Design review of the part built by this model. Coordinates are the model's own, in mm. Face numbers are marked on the shaded views. A direction names the side the tool comes from. Give positions to 0.01 mm unless a question says otherwise; leave off trailing zeros. Write each loop counter-clockwise with the first axis right and the second up, starting at its lowest first coordinate (ties: lowest second). Pieces come first, ordered by that corner, then holes. Notation, with made-up numbers: (71.5, 31) -> (129.5, 31) arc R14 ccw to (129.5, 45) -> close; hole circle Ø7 at (-13, 36.25). An arc over 180 degrees is marked (long way). Answer as a JSON object with one key per item and string values.
```python
from build123d import *

# Parameters (mm, degrees)
SKETCH1_R           = 1.65
BOSS_EXTRUDE1_DEPTH = 5
FILLET2_R           = 0.25
CUT_EXTRUDE1_DEPTH  = 4


with BuildPart() as part:
    # Sketch1 → Boss-Extrude1 (new body)
    # profile 1 of 2: a face of its own
    with BuildSketch(Plane.XY):
        with BuildLine():
            Line((-5.168635154, -1.464478016), (-25.218635154, -1.464478016))
            ThreePointArc((-25.218635154, -1.464478016), (-30.218635154, -6.464478016), (-25.218635154, -11.464478016))
            Line((-25.218635154, -11.464478016), (-3.218635154, -11.464478016))
            Line((-3.218635154, -11.464478016), (1.36555506, -4.468181425))
            ThreePointArc((1.36555506, -4.468181425), (-0.47833252, -2.282284635), (-3.218635154, -1.464478016))
            Line((-3.218635154, -1.464478016), (-5.168635154, -1.464478016))
        make_face()
        with Locations((-25.218635154, -6.464478016)):
            Circle(SKETCH1_R, mode=Mode.SUBTRACT)
        with Locations((-3.197929879, -6.257635448)):
            Circle(SKETCH1_R, mode=Mode.SUBTRACT)
    # profile 2 of 2: a face of its own
    with BuildSketch(Plane.XY):
        with BuildLine():
            Line((35.988446, 15.45724385), (-5.168635154, -1.464478016))
            Line((-5.168635154, -1.464478016), (-3.218635154, -1.464478016))
            ThreePointArc((-3.218635154, -1.464478016), (-0.47833252, -2.282284635), (1.36555506, -4.468181425))
            Line((1.36555506, -4.468181425), (29.450627286, 6.742809526))
            Line((29.450627286, 6.742809526), (35.767904523, 4.15974363))
            Line((35.767904523, 4.15974363), (36.563833051, 3.839605387))
            Line((36.563833051, 3.839605387), (45.016686804, 7.962377757))
            Line((45.016686804, 7.962377757), (43.305501447, 12.124329784))
            Line((43.305501447, 12.124329784), (35.988446, 15.45724385))
        make_face()
    extrude(amount=BOSS_EXTRUDE1_DEPTH)

    # Fillet2
    fillet2_edges = [part.edges().sort_by_distance(p)[0] for p in [
        (-14.218635154, -11.464478016, 0),
        (-30.218635154, -6.464478016, 0),
        (-15.193635154, -1.464478016, 0),
        (15.409905423, 6.996382917, 0),
        (-0.926540047, -7.966329721, 5),
        (39.646973723, 13.790786817, 0),
        (44.161094126, 10.04335377, 0),
        (40.790259928, 5.900991572, 0),
        (36.165868787, 3.999674508, 0),
        (32.609265904, 5.451276578, 0),
        (15.408091173, 1.137314051, 0),
        (-0.926540047, -7.966329721, 0),
        (15.408091173, 1.137314051, 5),
        (-3.218635154, -11.464478016, 2.5),
        (-5.168635154, -1.464478016, 2.5),
        (35.988446, 15.45724385, 2.5),
        (43.305501447, 12.124329784, 2.5),
        (45.016686804, 7.962377757, 2.5),
        (36.563833051, 3.839605387, 2.5),
        (35.767904523, 4.15974363, 2.5),
        (29.450627286, 6.742809526, 2.5),
        (1.36555506, -4.468181425, 2.5),
        (32.609265904, 5.451276578, 5),
        (36.165868787, 3.999674508, 5),
        (40.790259928, 5.900991572, 5),
        (44.161094126, 10.04335377, 5),
        (39.646973723, 13.790786817, 5),
        (15.409905423, 6.996382917, 5),
        (-15.193635154, -1.464478016, 5),
        (-30.218635154, -6.464478016, 5),
        (-14.218635154, -11.464478016, 5),
    ]]
    fillet(fillet2_edges, radius=FILLET2_R)

    # Sketch2 → Cut-Extrude1 (cut)
    with BuildSketch(Plane.XY):
        Polygon((-23.630921913, -9.214478016), (-22.043208673, -6.464478016), (-23.630921913, -3.714478016), (-26.806348394, -3.714478016), (-28.394061634, -6.464478016), (-26.806348394, -9.214478016), align=None)
        Polygon((-0.027560565, -6.436777135), (-1.45760397, -3.601585926), (-4.627973284, -3.422444239), (-6.368299193, -6.078493761), (-4.938255788, -8.91368497), (-1.767886474, -9.092826657), align=None)
    extrude(amount=CUT_EXTRUDE1_DEPTH, mode=Mode.SUBTRACT)


solid = part.part
```
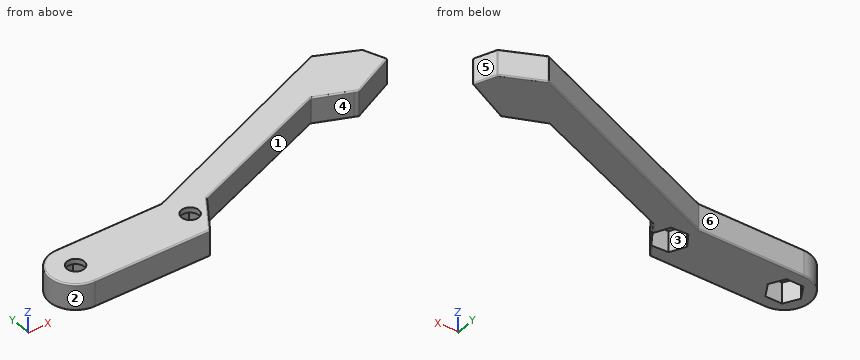
(1) We need section B-B, the plane x = -13. State the section outline as (y, z) points.
Here are the results:
{"outline": "(-11.46, 0.25) arc R0.25 ccw to (-11.21, 0) -> (-1.71, 0) arc R0.25 ccw to (-1.46, 0.25) -> (-1.46, 4.75) arc R0.25 ccw to (-1.71, 5) -> (-11.21, 5) arc R0.25 ccw to (-11.46, 4.75) -> close"}
(2) Clearance check with flat-ended pins moving along their axes: pin 1 (3 mm diameter, centred on x = 18.5, z = 2.5, fed in from -Y); pin 2 (1 mm diameter, centred on x = -25.5, z = 1.5, fed in from +Y). State where each tip first meets the part, or that it passes through.
Here are the results:
{"pin 1": "stops at y = 1.77", "pin 2": "stops at y = -1.46"}
(3) The part is to be moulded in two halves that separate along X. For the marked faces 4, 5 and 6, say which applies: +X half, -X half, draft (parallel to the pull), parting line (faces both ways), or undercut.
Here are the results:
{"face 4": "undercut", "face 5": "+X half", "face 6": "draft"}
(4) We need section A-A, the plane z = 1.8. Give the number of separate pieces and of enclosed holes in the cut face, then the cut area to 3 significant figures.
Here are the results:
{"separate pieces": "1", "enclosed holes": "2", "area": "533 mm²"}
(5) For line 1 along X through (y, z) = (-6.25, 0.3); line 2 along Y through (x, z) = (-15, 4.5); line 3 along Y through (x, z) = (-27, 2.65), list the stretches that pass through material, from the lowest coordinate up.
Here are the results:
{"line 1": "x = -30.21 to -28.27, -22.17 to -6.28, -0.12 to 0.2", "line 2": "y = -11.46 to -1.46", "line 3": "y = -11.14 to -8.88, -4.05 to -1.79"}
(6) For the marked faces 1, 2 and 3, list the 3-axis set-ups (+Z, -Z, +X, -X, +Y, -Y) from which the entire face can be reached by the end or side of a thin tool; tool diameter is ignored.
Here are the results:
{"face 1": "+Z, -Z, -Y", "face 2": "+Z, -Z, -X", "face 3": "-Z"}
